Geometry: see drawing. Coordinates: mm, zero at the bounding-box minimum. Coordinates: 2 decimals unless noted, no trailing zeros. Write each loop counter-clockwise with the first axis right and the second up, starting at its lowest first coordinate (ties: lowest second). Pieces come first, ordered by that corner, then holes. Notation, with made-up numbers: (49.25, -8) - (80.25, -8) arc R27 ccw to (80.25, 24) - close; hole circle Ø2 at (59, 84.25). An arc over 180 degrees is marked (long way). One line per question, with ' | ' between items. Start each with the question number.
1) Section query D-D on z = 7.5. Return loops of the section in (x, y), and give its area (3 significant figures).
2) Section query C-C on y = 3. Return loops of the section in (x, z).
3) Section query B-B on x = 30.5. Return loops of the section in (y, z), and give its area (3 significant figures).
4) Line query: line 1 (X direction, y = 1.5, z = 10); line 2 (X direction, y = 5.5, z = 8.75); line 3 (Z direction, x = 2.5, y = 2.5). Output: solid intervals per line, ascending.
5) Section query A-A on z = 2. Return loops of the section in (x, y).
6) First-contact query: P1, Ø4, axis at x = 74.5, z = 7, coming from the -Y side; P2, Ø1.6, axis at y = 0.5, z = 11.5, coming from the +X side; P3, Ø1.9, axis at x = 89, y = 2, coming from the -Z side. Flat tips, straight axial feed; report the tip coordinate or a pass-through.
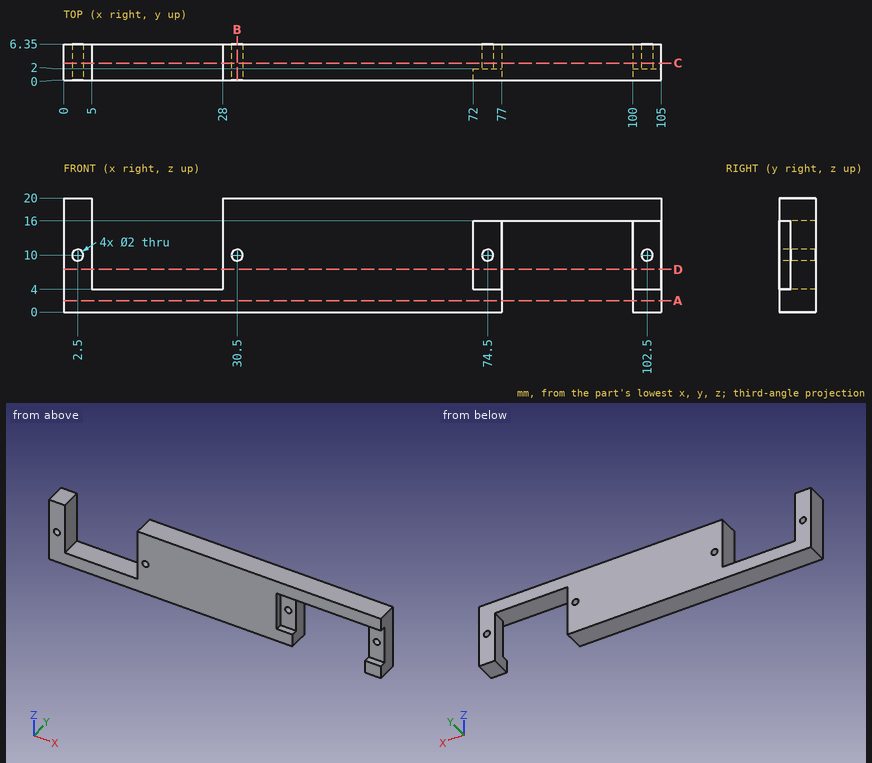
Answer key:
1) outline: (0, 0) - (5, 0) - (5, 6.35) - (0, 6.35) - close; (28, 0) - (72, 0) - (72, 2) - (77, 2) - (77, 6.35) - (28, 6.35) - close; (100, 2) - (105, 2) - (105, 6.35) - (100, 6.35) - close | area: 355 mm²
2) outline: (0, 0) - (77, 0) - (77, 16) - (100, 16) - (100, 0) - (105, 0) - (105, 20) - (28, 20) - (28, 4) - (5, 4) - (5, 20) - (0, 20) - close; hole circle Ø2 at (2.5, 10); hole circle Ø2 at (30.5, 10); hole circle Ø2 at (74.5, 10); hole circle Ø2 at (102.5, 10)
3) outline: (0, 0) - (6.35, 0) - (6.35, 9) - (0, 9) - close; (0, 11) - (6.35, 11) - (6.35, 20) - (0, 20) - close | area: 114 mm²
4) line 1: 0 to 1.5, 3.5 to 5, 28 to 29.5, 31.5 to 72 | line 2: 0 to 5, 28 to 77, 100 to 105 | line 3: 0 to 9, 11 to 20
5) outline: (0, 0) - (77, 0) - (77, 6.35) - (0, 6.35) - close; (100, 0) - (105, 0) - (105, 6.35) - (100, 6.35) - close
6) P1: y = 2 | P2: x = 72 | P3: z = 16
